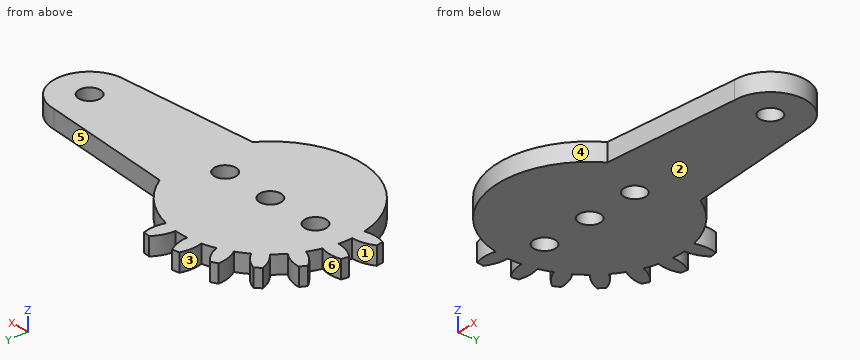
from build123d import *

# Parameters (mm, degrees)
SKETCH1_R           = 1.5
BOSS_EXTRUDE1_DEPTH = 2.5


with BuildPart() as part:
    # Sketch1 → Boss-Extrude1 (new body)
    with BuildSketch(Plane.XY):
        with BuildLine():
            Line((30, 5), (10.663780267, 6.521793497))
            ThreePointArc((10.663780267, 6.521793497), (7.359278279, 10.104010254), (2.936071308, 12.150287456))
            ThreePointArc((2.936071308, 12.150287456), (3.170504769, 13.6920006), (2.918578378, 15.230952047))
            Line((2.918578378, 15.230952047), (1.930890038, 15.387386512))
            ThreePointArc((1.930890038, 15.387386512), (1.215731652, 14.001606246), (0.962275561, 12.462905991))
            ThreePointArc((0.962275561, 12.462905991), (0, 12.5), (-0.962275561, 12.462905991))
            ThreePointArc((-0.962275561, 12.462905991), (-1.215731652, 14.001606246), (-1.930890038, 15.387386512))
            Line((-1.930890038, 15.387386512), (-2.918578378, 15.230952047))
            ThreePointArc((-2.918578378, 15.230952047), (-3.170504769, 13.6920006), (-2.936071308, 12.150287456))
            ThreePointArc((-2.936071308, 12.150287456), (-3.86271243, 11.888206454), (-4.766428193, 11.555568453))
            ThreePointArc((-4.766428193, 11.555568453), (-5.482963788, 12.940637118), (-6.591349484, 14.037596375))
            Line((-6.591349484, 14.037596375), (-7.482356008, 13.583605875))
            ThreePointArc((-7.482356008, 13.583605875), (-7.246390093, 12.042126537), (-6.54701506, 10.648314129))
            ThreePointArc((-6.54701506, 10.648314129), (-7.347315654, 10.11271243), (-8.104009624, 9.517091363))
            ThreePointArc((-8.104009624, 9.517091363), (-9.213485226, 10.612948266), (-10.606601718, 11.313708499))
            Line((-10.606601718, 11.313708499), (-11.313708499, 10.606601718))
            ThreePointArc((-11.313708499, 10.606601718), (-10.612948266, 9.213485226), (-9.517091363, 8.104009624))
            ThreePointArc((-9.517091363, 8.104009624), (-10.11271243, 7.347315654), (-10.648314129, 6.54701506))
            ThreePointArc((-10.648314129, 6.54701506), (-12.042126537, 7.246390093), (-13.583605875, 7.482356008))
            Line((-13.583605875, 7.482356008), (-14.037596375, 6.591349484))
            ThreePointArc((-14.037596375, 6.591349484), (-12.940637118, 5.482963788), (-11.555568453, 4.766428193))
            ThreePointArc((-11.555568453, 4.766428193), (-11.888206454, 3.86271243), (-12.150287456, 2.936071308))
            ThreePointArc((-12.150287456, 2.936071308), (-13.6920006, 3.170504769), (-15.230952047, 2.918578378))
            Line((-15.230952047, 2.918578378), (-15.387386512, 1.930890038))
            ThreePointArc((-15.387386512, 1.930890038), (-14.001606246, 1.215731652), (-12.462905991, 0.962275561))
            ThreePointArc((-12.462905991, 0.962275561), (-12.5, 0), (-12.462905991, -0.962275561))
            ThreePointArc((-12.462905991, -0.962275561), (-14.001606246, -1.215731652), (-15.387386512, -1.930890038))
            Line((-15.387386512, -1.930890038), (-15.230952047, -2.918578378))
            ThreePointArc((-15.230952047, -2.918578378), (-13.6920006, -3.170504769), (-12.150287456, -2.936071308))
            ThreePointArc((-12.150287456, -2.936071308), (-1.940818593, -12.348409743), (10.663780267, -6.521793497))
            Line((10.663780267, -6.521793497), (30, -5))
            ThreePointArc((30, -5), (35, 0), (30, 5))
        make_face()
        with Locations((30, 0)):
            Circle(SKETCH1_R, mode=Mode.SUBTRACT)
        Circle(SKETCH1_R, mode=Mode.SUBTRACT)
        with Locations((-7.5, 0)):
            Circle(SKETCH1_R, mode=Mode.SUBTRACT)
        with Locations(Location((7.5, 0, 0), (0, 0, 180))):
            Circle(SKETCH1_R, mode=Mode.SUBTRACT)
    extrude(amount=BOSS_EXTRUDE1_DEPTH)


solid = part.part
Build history of the part. All positions in model axes, mm. Face numbers are marked on the shaded views. A direction names the side the tool comes from. Round coordinates to 2 decimals unless told otherwise and drop trailing zeros. Loops run counter-clockwise (first coordinate to the right, second up) from the corner with the lowest first, then second, coordinate; pieces in that order, holes last. Notation, with made-up numbers: (76.25, -5.75) -> (98.25, -5.75) arc R28 cw to (98.25, 27.25) -> close; hole circle Ø1 at (24.5, 39). An arc over 180 degrees is marked (long way). One line per item, written item: value. Start each with the question number.
Q1. Cut at A-A on x = 7.5. List the corners of the cut face in (y, z).
Q2. Drop a flat-ended pin along its axis: pin 1 Ø1 at (y, z) = (9.5, 2) entering from -X. Give the stop position or say it passes through.
Q3. 3-axis set-ups, long thin cutter, end or side, ignore diameter. For the marked faces 1, 2 and 3: which of +Z, -Z, +X, -X, +Y, -Y reach the whole face in a straight line?
Q4. Cut at D-D on z = 1. Count the separate pieces of the cut face and the enclosed holes in it, plus the area to 3 significant figures.
Q5. Probe line 1 along Y through (x, z) = (0, 1.7); line 2 along Y through (x, z) = (30, 0.75); line 3 along X through (y, z) = (12.75, 2.1). List the from-to ranges inside material, lowest first.
Q6. Two-plate mould, pull along Y, no slides. Class the marked faces 4, 5 and 6: released by +Y, released by -Y, zero draft, split by the parting line, or undercut.
Q7. Cut at B-B on y = 0. List the corners of the cut face in (x, z), plus the area to 4 significant figures.
Q8. Cut at C-C on x = 0. List the corners of the cut face in (y, z), plus the area to 3 significant figures.
Computed:
1. outline: (-10, 0) -> (-1.5, 0) -> (-1.5, 2.5) -> (-10, 2.5) -> close; (1.5, 0) -> (10, 0) -> (10, 2.5) -> (1.5, 2.5) -> close
2. pin 1: x = -11.08
3. face 1: +Z, -Z, -X
3. face 2: -Z, +X, -X, +Y, -Y
3. face 3: +Z, -Z
4. separate pieces: 1
4. enclosed holes: 4
4. area: 747 mm²
5. line 1: -12.5 to -1.5, 1.5 to 12.5
5. line 2: -5 to -1.5, 1.5 to 5
5. line 3: -7.42 to -5.35, -3.09 to -0.97, 0.97 to 3.09
6. face 4: released by -Y
6. face 5: released by +Y
6. face 6: undercut
7. outline: (-12.5, 0) -> (-9, 0) -> (-9, 2.5) -> (-12.5, 2.5) -> close; (-6, 0) -> (-1.5, 0) -> (-1.5, 2.5) -> (-6, 2.5) -> close; (1.5, 0) -> (6, 0) -> (6, 2.5) -> (1.5, 2.5) -> close; (9, 0) -> (28.5, 0) -> (28.5, 2.5) -> (9, 2.5) -> close; (31.5, 0) -> (35, 0) -> (35, 2.5) -> (31.5, 2.5) -> close
7. area: 88.75 mm²
8. outline: (-12.5, 0) -> (-1.5, 0) -> (-1.5, 2.5) -> (-12.5, 2.5) -> close; (1.5, 0) -> (12.5, 0) -> (12.5, 2.5) -> (1.5, 2.5) -> close
8. area: 55.0 mm²
